Source: CAD feature listing. Evaluate the final solid. Frame: model axes, mm. A direction names the side the tool comes from. Coordinates: 2 decimals unless noted, no trailing zeros. Loops run counter-clockwise (first coordinate to the right, second up) from the corner with the lowest first, then second, coordinate; pieces in that order, holes last. Notation, with made-up numbers: (-15.75, 83) - (27.25, 83) arc R20 ccw to (27.25, 116) - close; hole circle Ø11 at (33.25, -7.5). An arc over 180 degrees is marked (long way). Use one line per item in the form item = value. Start each with the question number.
Autodesk Inventor part; units mm, degrees
ref_plane "YZ Plane" through (0, 0, 0) normal (1, 0, 0) x (0, 1, 0)
ref_plane "XZ Plane" through (0, 0, 0) normal (0, 1, 0) x (-1, 0, 0)
ref_plane "XY Plane" through (0, 0, 0) normal (0, 0, 1) x (1, 0, 0)
sketch "Sketch1" plane through (0, 0, 0) normal (0, 0, 1) x (1, 0, 0)
  line L0 (0, 0) -> (11, 0)
  line L1 (11, 0) -> (11, 45)
  line L2 (11, 45) -> (0, 45)
  line L3 (0, 45) -> (0, 0)
  line L4 (0, 22.5) -> (11, 22.5) construction
  line L5 (11, 35) -> (12.7, 35)
  line L6 (12.7, 35) -> (12.7, 10)
  line L7 (12.7, 10) -> (11, 10)
  line L8 (11, 10) -> (11, 35)
  dimension "d0" = 11
  dimension "d1" = 45
  dimension "d2" = 1.7
  dimension "d3" = 25
extrude "Extrusion1" add sketch "Sketch1" along normal blind 401
properties part number "prowadnica 400mm pelny wysuw"
(1) Contact query for flat-ended pins moving along their axis: pin 1 (6 mm diameter, centred on x = 5, y = 36.5, fed in from -Z); pin 2 (1.4 mm diameter, centred on x = 12, z = 179.5, fed in from -Y); pin 3 (3 mm diameter, centred on y = 4.5, z = 195, fed in from +X); pin 4 (1.9 mm diameter, centred on x = 12, z = 110, fed in from +Y). Output: stop coordinate, or through.
(2) Material intervals for line 1 (X direction, y = 4.5, z = 110.5); line 2 (Y direction, x = 11.75, z = 96.5), sorted ascending.
(3) Cut plane A-A, the plane z = 174.5. Output: boundary loops of the cut face in (x, y), plus the area to 4 significant figures.
(4) Access query for faces 1 (the face through (11, 5, 198)), 2 (the face through (5, 0, 198)), 3 (the face through (11, 40, 198)). Directions: +Z, -Z, +X, -X, +Y, -Y. A direction counts if a zero-diameter tool reaches every point of the face in a straight line with its end or side. Return the directions, or none.
Recorded:
q1.pin_1 = 0
q1.pin_2 = 10
q1.pin_3 = 11
q1.pin_4 = 35
q2.line_1 = 0 to 11
q2.line_2 = 10 to 35
q3.outline = (0, 0) - (11, 0) - (11, 10) - (12.7, 10) - (12.7, 35) - (11, 35) - (11, 45) - (0, 45) - close
q3.area = 537.5 mm²
q4.face_1 = +Z, -Z, +X, -Y
q4.face_2 = +Z, -Z, +X, -X, -Y
q4.face_3 = +Z, -Z, +X, +Y
